Could you check a few things on this model? Use its own coordinates, in mm. Give positions to 0.01 mm unless a question says otherwise; leave off trailing zeros. Order: outer loops, then holes, each group sorted by start corner. A loop starts at its lowest first (then second) coordinate and runs counter-clockwise, first axis right, second up.
from build123d import *

# Parameters (mm, degrees)
BOSS_EXTRUDE1_DEPTH         = 1143
F_1_4_0_25_DIAMETER_HOLE1_D = 6.35
FILLET2_R                   = 3.175


with BuildPart() as part:
    # Sketch1 → Boss-Extrude1 (new body)
    with BuildSketch(Plane(origin=(0, 0, 0), x_dir=(1, 0, 0), z_dir=(0, 1, 0))):
        Polygon((-44.45, 19.05), (-37.731942035, -19.05), (44.45, -19.05), (44.45, 19.05), align=None)
    extrude(amount=BOSS_EXTRUDE1_DEPTH)

    # 1/4 (0.25) Diameter Hole1 (through all)
    with Locations(Plane(origin=(0, 0, 19.05), x_dir=(-1, 0, 0), z_dir=(0, 0, 1))):
        with Locations((-8.817444165, -52.3875), (-8.817444165, -398.4625), (-8.817444165, -744.5375), (-8.817444165, -1090.6125)):
            Hole(F_1_4_0_25_DIAMETER_HOLE1_D / 2)

    # Fillet2
    fillet2_edges = [part.edges().sort_by_distance(p)[0] for p in [
        (44.45, 571.5, -19.05),
        (44.45, 571.5, 19.05),
    ]]
    fillet(fillet2_edges, radius=FILLET2_R)


solid = part.part
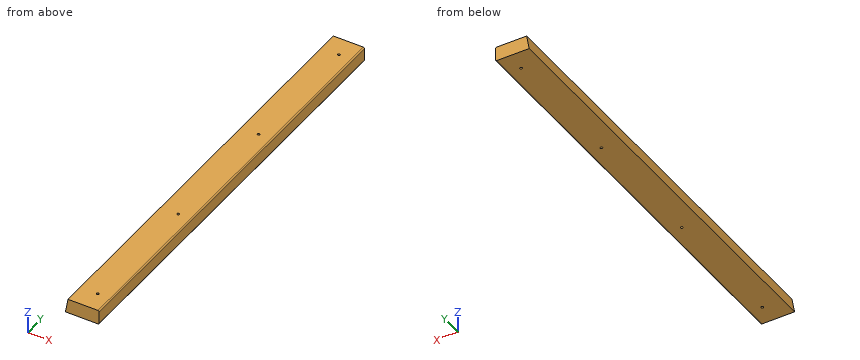
Item 1: Please list where these lines run through material, in increasing order: line 1 along Y through (x, z) = (8.5, 16); line 2 along Y through (x, z) = (10.5, 6.5); line 3 along X through (y, z) = (351.5, -8.5).
Findings:
line 1: y = 0 to 49.23, 55.55 to 395.3, 401.62 to 741.38, 747.7 to 1087.45, 1093.77 to 1143
line 2: y = 0 to 49.69, 55.08 to 395.77, 401.16 to 741.84, 747.23 to 1087.92, 1093.31 to 1143
line 3: x = -42.59 to 44.45
Item 2: For pin 1 (5.5 mm diameter, centred on x = 8.82, y = 52.39, fed in from -Z); pin 2 (10 mm diameter, centred on y = 375, z = -6, fed in from -X); pin 3 (3 mm diameter, centred on y = 789.5, z = 8, fed in from -X); pin 4 (1 mm diameter, centred on y = 708.5, z = 5.5, fed in from -X), each with a flat end and sliding along its axis, tell me the tip position at first contact or that it passes through.
Findings:
pin 1: passes through
pin 2: stops at x = -43.03
pin 3: stops at x = -39.94
pin 4: stops at x = -40.21
Item 3: Imagine slicing it at B-B on y = 468. List the corners of the cut face in (x, z) for me (3 decimals), then the cut area to 3 significant figures.
Findings:
outline: (-44.45, -19.05) - (41.275, -19.05) arc R3.175 ccw to (44.45, -15.875) - (44.45, 15.875) arc R3.175 ccw to (41.275, 19.05) - (-37.732, 19.05) - close
area: 3,250 mm2
Item 4: Imagine slicing it at A-A on z = -7.5. Give the number of separate pieces and of enclosed holes in the cut face, then the cut area to 3 significant figures.
Findings:
separate pieces: 1
enclosed holes: 4
area: 99,200 mm2
